Autodesk Inventor part; units mm, degrees
ref_plane "YZ Plane" through (0, 0, 0) normal (1, 0, 0) x (0, 1, 0)
ref_plane "XZ Plane" through (0, 0, 0) normal (0, 1, 0) x (-1, 0, 0)
ref_plane "XY Plane" through (0, 0, 0) normal (0, 0, 1) x (1, 0, 0)
sketch "草图1" plane through (0, 0, 0) normal (0, 0, 1) x (1, 0, 0)
  line L0 (-40, 25) -> (40, 25)
  line L1 (40, 25) -> (40, -25)
  line L2 (40, -25) -> (-40, -25)
  line L3 (-40, 25) -> (40, -25) construction
  line L4 (40, 25) -> (-40, -25) construction
  arc A0 (-40, 25) -> (-40, -25) centre (-40, 0) ccw
  circle A1 centre (-40, 0) radius 15
  line L5 (-39.6714, -125) -> (39.6714, -125)
  line L6 (39.6714, -125) -> (39.6714, -75)
  line L7 (39.6714, -75) -> (-39.6714, -75)
  line L8 (-39.6714, -125) -> (39.6714, -75) construction
  line L9 (39.6714, -125) -> (-39.6714, -75) construction
  arc A2 (-39.6714, -75) -> (-39.6714, -125) centre (-40, -100) ccw
  circle A3 centre (-40, -100) radius 15
  point P0 (0, 0)
  point P1 (0, -100)
  dimension "d0" = 50
  dimension "d3" = 30
  dimension "d11" = 50
  dimension "d12" = 30
  dimension "d13" = 100
  dimension "d14" = 0
  dimension "d15" = 25
  dimension "d16" = 80
extrude "拉伸1" add sketch "草图1" along normal mid plane 100
sketch "草图2" plane through (-40, 25, 50) normal (0, 1, 0) x (1, 0, 0)
  line L0 (40, 50) -> (0, 50)
  line L1 (0, 100) -> (0, 0)
  line L2 (50, 85) -> (-98.1355, 85)
  line L3 (-98.1355, 85) -> (-98.1355, 15)
  line L4 (-98.1355, 15) -> (50, 15)
  line L5 (50, 15) -> (50, 85)
  line L6 (50, 85) -> (-98.1355, 15) construction
  line L7 (-98.1355, 85) -> (50, 15) construction
  line L8 (80, 0) -> (80, 100)
  point P0 (-24.0677, 50)
  dimension "d4" = 30
  dimension "d5" = 70
extrude "拉伸2" cut sketch "草图2" against normal through all
sketch "草图3" plane through (40, -25, 50) normal (1, 0, 0) x (0, 0, -1)
  line L0 (100, 50) -> (0, 50)
  line L1 (0, 50) -> (100, 50)
  line L2 (100, 50) -> (100, -100)
  line L3 (100, -100) -> (0, -100)
  line L4 (0, -100) -> (0, 50)
  point P0 (50, 25)
  point P1 (15, 50)
  dimension "d8" = 150
extrude "拉伸3" add sketch "草图3" against normal blind 30
sketch "草图4" plane through (40, -125, 50) normal (1, 0, 0) x (0, 0, -1)
  line L0 (100, 100) -> (100, 50)
  line L1 (100, 75) -> (0, 75)
  line L2 (0, 0) -> (0, 150)
  line L3 (15, 0) -> (85, 0)
  line L4 (50, 0) -> (50, 150)
  line L5 (0, 150) -> (100, 150)
  circle A0 centre (50, 75) radius 75
  point P0 (50, 125)
extrude "拉伸4" add sketch "草图4" along normal blind 30 contours L4 A0 L2 L1 | L4 A0 | L1 L2 A0 L4 | L2 A0
sketch "草图5" plane through (70, -50, 0) normal (1, 0, 0) x (0, 0, -1)
  circle A0 centre (0, 0) radius 30
  point P0 (0, 50)
  dimension "d19" = 60
extrude "拉伸5" cut sketch "草图5" against normal blind 15
properties part number "Wrist" material "钢，高强度，低合金"
Geometry check sheet. Reference: the model listing, model coordinates, mm. A direction names the side the tool comes from. Give positions to 0.01 mm unless a question says otherwise; leave off trailing zeros. Order: outer loops, then holes, each group sorted by start corner. A loop starts at its lowest first (then second) coordinate and runs counter-clockwise, first axis right, second up.
1. Thickness scan on L1, parallel to Y at x = -40, z = 44.5; L2, parallel to Z at x = -57, y = 6.5; L3, parallel to Y at x = -10.5, z = 40. Record the ranges inside material, lowest first.
2. Section check B-B, the plane z = -40. Enter the section's corners in (x, y).
3. Release check for a two-part mould opening along Z. For faces 1 (the face through (-64.996, -100.554, 42.395)), 2 (the face through (55, -50, 0)), 3 (the face through (22, -49, 50)) record: pulls with the +Z half, pulls with the -Z half, needs draft (parallel to the pull), parting line crosses it, or undercut.
4. Access from +Z, -Z, +X, -X, +Y, -Y to the whole of each face (thin tool, end or side, straight path). Record for faces 4 (the face through (40, 19, -38)), 5 (the face through (62.605, -79.287, 6.503)), 6 (the face through (-20, -100, 35)), 7 (the face through (-15, -25, -43)), 8 (the face through (40, -49, -60)).
5. Section check C-C, the plane y = -100. Enter the section's corners in (x, z), and give its area (3 significant figures).
6. Section check D-D, the plane z = 19.5. Enter the section's corners in (x, y).
7. Gauge pin test, flat ends, axial feed: pin 1 Ø1 at (x, y) = (-16, -21) entering from +Z; pin 2 Ø8 at (y, z) = (-71.5, -59.5) entering from -X; pin 3 Ø1 at (x, y) = (48, -66) entering from +Z. Record the tip position at first contact, or that the pin passes through.
8. Section check A-A, the plane x = 5. Enter the section's corners in (y, z).
Values follow:
1. L1: y = -125 to -115, -85 to -75, -25 to -15, 15 to 25
1. L2: z = -50 to -35, 35 to 50
1. L3: y = -125 to -75, -25 to 25
2. outline: (-40, -25) - (10, -25) - (10, -75) - (-39.67, -75) arc R25 ccw (long way) to (-39.67, -125) - (40, -125) - (40, -113.44) - (70, -113.44) - (70, 13.44) - (40, 13.44) - (40, 25) - (-40, 25) arc R25 ccw to start; hole circle Ø30 at (-40, -100); hole circle Ø30 at (-40, 0)
3. face 1: needs draft
3. face 2: undercut
3. face 3: pulls with the +Z half
4. face 4: -Z, +X, +Y
4. face 5: +X
4. face 6: -X, +Y, -Y
4. face 7: +Z, -Z, -X
4. face 8: -Z, -X, +Y, -Y
5. outline: (-65, -50) - (-55, -50) - (-55, -35) - (-65, -35) - close; (-65, 35) - (-55, 35) - (-55, 50) - (-65, 50) - close; (-25, -50) - (40, -50) - (40, -55.9) - (70, -55.9) - (70, 55.9) - (40, 55.9) - (40, 50) - (-25, 50) - (-25, 35) - (10, 35) - (10, -35) - (-25, -35) - close
5. area: 7,700 mm2
6. outline: (10, -125) - (40, -125) - (40, -122.42) - (70, -122.42) - (70, -72.8) - (55, -72.8) - (55, -27.2) - (70, -27.2) - (70, 22.42) - (40, 22.42) - (40, 25) - (10, 25) - close
7. pin 1: stops at z = 50
7. pin 2: stops at x = 40
7. pin 3: stops at z = 73.38
8. outline: (-125, -50) - (-75, -50) - (-75, -35) - (-125, -35) - close; (-125, 35) - (-75, 35) - (-75, 50) - (-125, 50) - close; (-25, -50) - (25, -50) - (25, -35) - (-25, -35) - close; (-25, 35) - (25, 35) - (25, 50) - (-25, 50) - close
